Work out the finished part from the listing and answer in its coordinate system (mm). A direction names the side the tool comes from. Give positions to 0.01 mm unless a question says otherwise; leave off trailing zeros. Order: outer loops, then holes, each group sorted by start corner. A loop starts at its lowest first (then second) coordinate and runs counter-clockwise, first axis right, second up.
```python
from build123d import *

# Parameters (mm, degrees)
SKETCH001_W     = 100
SKETCH001_H     = 132
PAD_DEPTH       = 2.5
SKETCH002_R     = 3.5
SKETCH002_R_2   = 1.75
PAD001_DEPTH    = 4
PAD002_DEPTH    = 2.5
SKETCH004_R     = 3
HOLE_DEPTH      = 25
CHAMFER_1_ANGLE = 49
CHAMFER_1_SIZE  = 1
CHAMFER_2_ANGLE = 49
CHAMFER_2_SIZE  = 1
CHAMFER_3_ANGLE = 49
CHAMFER_3_SIZE  = 1
CHAMFER_4_ANGLE = 49
CHAMFER_4_SIZE  = 1
SKETCH005_W     = 10
SKETCH005_H     = 5
PAD003_DEPTH    = 12.5
FILLET_R        = 3.5
FILLET001_R     = 0.75


with BuildPart() as part:
    # Sketch001 → Pad (new body)
    with BuildSketch(Plane.XY):
        with Locations((50, 66)):
            Rectangle(SKETCH001_W, SKETCH001_H)
    extrude(amount=PAD_DEPTH)

    # Sketch002 (on Face6 of Pad) → Pad001 (join)
    with BuildSketch(Plane.XY.offset(2.5)):
        with Locations((76.5, 10)):
            Circle(SKETCH002_R)
        with Locations((76.5, 10)):
            Circle(SKETCH002_R_2, mode=Mode.SUBTRACT)
        with Locations((18.5, 10)):
            Circle(SKETCH002_R)
        with Locations((18.5, 10)):
            Circle(SKETCH002_R_2, mode=Mode.SUBTRACT)
        with Locations((18.5, 59)):
            Circle(SKETCH002_R)
        with Locations((18.5, 59)):
            Circle(SKETCH002_R_2, mode=Mode.SUBTRACT)
        with Locations((76.5, 59)):
            Circle(SKETCH002_R)
        with Locations((76.5, 59)):
            Circle(SKETCH002_R_2, mode=Mode.SUBTRACT)
        with Locations((87.1, 77.3)):
            Circle(SKETCH002_R)
        with Locations((87.1, 77.3)):
            Circle(SKETCH002_R_2, mode=Mode.SUBTRACT)
        with Locations((17.5, 77.3)):
            Circle(SKETCH002_R)
        with Locations((17.5, 77.3)):
            Circle(SKETCH002_R_2, mode=Mode.SUBTRACT)
        with Locations((17.5, 121.3)):
            Circle(SKETCH002_R)
        with Locations((17.5, 121.3)):
            Circle(SKETCH002_R_2, mode=Mode.SUBTRACT)
        with Locations((87.1, 121.3)):
            Circle(SKETCH002_R)
        with Locations((87.1, 121.3)):
            Circle(SKETCH002_R_2, mode=Mode.SUBTRACT)
    extrude(amount=PAD001_DEPTH)

    # Sketch003 → Pad002 (join)
    with BuildSketch(Plane.XY):
        with BuildLine():
            Line((-7.5, 102), (0, 102))
            Line((0, 102), (0, 87))
            Line((0, 87), (-7.5, 87))
            ThreePointArc((-7.5, 102), (-15.00002, 94.5), (-7.5, 87))
        make_face()
        with BuildLine():
            Line((-7.5, 45), (0, 45))
            Line((0, 45), (0, 30))
            Line((0, 30), (-7.5, 30))
            ThreePointArc((-7.5, 45), (-15.00002, 37.5), (-7.5, 30))
        make_face()
        with BuildLine():
            Line((100, 102), (107.5, 102))
            ThreePointArc((107.5, 87), (114.99998, 94.5), (107.5, 102))
            Line((107.5, 87), (100, 87))
            Line((100, 87), (100, 102))
        make_face()
        with BuildLine():
            Line((100, 45), (107.5, 45))
            ThreePointArc((107.5, 30), (114.99998, 37.5), (107.5, 45))
            Line((107.5, 30), (100, 30))
            Line((100, 30), (100, 45))
        make_face()
    extrude(amount=PAD002_DEPTH)

    # Sketch004 (on Face18 of Pad002) → Hole (cut)
    with BuildSketch(Plane.XY.offset(2.5)):
        with Locations((-7.5, 94.5)):
            Circle(SKETCH004_R)
        with Locations((107.5, 94.5)):
            Circle(SKETCH004_R)
        with Locations((107.5, 37.5)):
            Circle(SKETCH004_R)
        with Locations((-7.5, 37.5)):
            Circle(SKETCH004_R)
    extrude(amount=-HOLE_DEPTH, mode=Mode.SUBTRACT)

    # Chamfer 1
    chamfer_1_edges = [part.edges().sort_by_distance(p)[0] for p in [
        (104.5, 94.5, 2.5),
    ]]
    chamfer_1_side = part.faces().sort_by_distance((103.75, 87.212132, 2.5))[0]
    chamfer(chamfer_1_edges, length=CHAMFER_1_SIZE, angle=CHAMFER_1_ANGLE, reference=chamfer_1_side)

    # Chamfer 2
    chamfer_2_edges = [part.edges().sort_by_distance(p)[0] for p in [
        (104.5, 37.5, 2.5),
    ]]
    chamfer_2_side = part.faces().sort_by_distance((103.75, 30.212132, 2.5))[0]
    chamfer(chamfer_2_edges, length=CHAMFER_2_SIZE, angle=CHAMFER_2_ANGLE, reference=chamfer_2_side)

    # Chamfer 3
    chamfer_3_edges = [part.edges().sort_by_distance(p)[0] for p in [
        (-10.5, 37.5, 2.5),
    ]]
    chamfer_3_side = part.faces().sort_by_distance((-3.75, 44.787868, 2.5))[0]
    chamfer(chamfer_3_edges, length=CHAMFER_3_SIZE, angle=CHAMFER_3_ANGLE, reference=chamfer_3_side)

    # Chamfer 4
    chamfer_4_edges = [part.edges().sort_by_distance(p)[0] for p in [
        (-10.5, 94.5, 2.5),
    ]]
    chamfer_4_side = part.faces().sort_by_distance((-3.75, 101.787868, 2.5))[0]
    chamfer(chamfer_4_edges, length=CHAMFER_4_SIZE, angle=CHAMFER_4_ANGLE, reference=chamfer_4_side)

    # Sketch005 → Pad003 (join)
    with BuildSketch(Plane.XY):
        with Locations((-5, 66)):
            Rectangle(SKETCH005_W, SKETCH005_H)
        with Locations((-5, 76)):
            Rectangle(SKETCH005_W, SKETCH005_H)
        with Locations((-5, 56)):
            Rectangle(SKETCH005_W, SKETCH005_H)
    extrude(amount=PAD003_DEPTH)

    # Fillet
    fillet_edges = [part.edges().sort_by_distance(p)[0] for p in [
        (0, 56, 12.5),
        (-10, 56, 12.5),
        (-10, 66, 12.5),
        (0, 66, 12.5),
        (-10, 76, 12.5),
        (0, 76, 12.5),
    ]]
    fillet(fillet_edges, radius=FILLET_R)

    # Fillet001
    fillet001_edges = [part.edges().sort_by_distance(p)[0] for p in [
        (-5, 53.5, 12.5),
        (-5, 58.5, 12.5),
        (-5, 63.5, 12.5),
        (-5, 68.5, 12.5),
        (-5, 73.5, 12.5),
        (-5, 78.5, 12.5),
    ]]
    fillet(fillet001_edges, radius=FILLET001_R)


solid = part.part
```
1. The part is cut by section C-C (y = 10). Write down the section's boundary in (x, z).
Findings below:
outline: (0, 0) - (100, 0) - (100, 2.5) - (80, 2.5) - (80, 6.5) - (78.25, 6.5) - (78.25, 2.5) - (74.75, 2.5) - (74.75, 6.5) - (73, 6.5) - (73, 2.5) - (22, 2.5) - (22, 6.5) - (20.25, 6.5) - (20.25, 2.5) - (16.75, 2.5) - (16.75, 6.5) - (15, 6.5) - (15, 2.5) - (0, 2.5) - close
2. The mould has two halves that part along X. Classify faces 4 (the face through (-9, 56.02, 11.45)), 5 (the face through (-5, 53.5, 6)), 6 (the face through (-1, 56.02, 11.45)), 7 (the face through (0, 56, 6)): pulls with the +X half, pulls with the -X half, needs draft (parallel to the pull), parting line crosses it, or undercut.
Findings below:
face 4: pulls with the -X half
face 5: needs draft
face 6: pulls with the +X half
face 7: undercut
3. Straight lines are drawn through the part: probe 1 along Z at (x, y) = (8, 106); probe 2 along X at (y, z) = (75.5, 9.25); probe 3 along X at (y, z) = (13, 3). For each, find the intervals that lie inside material, in ascending order.
Findings below:
probe 1: z = 0 to 2.5
probe 2: x = -9.99 to -0.01
probe 3: x = 16.7 to 20.3, 74.7 to 78.3
4. The part is cut by section B-B (x = 76.5). Write down the section's boundary in (y, z), then the cut area to 3 significant figures.
Findings below:
outline: (0, 0) - (132, 0) - (132, 2.5) - (62.5, 2.5) - (62.5, 6.5) - (60.75, 6.5) - (60.75, 2.5) - (57.25, 2.5) - (57.25, 6.5) - (55.5, 6.5) - (55.5, 2.5) - (13.5, 2.5) - (13.5, 6.5) - (11.75, 6.5) - (11.75, 2.5) - (8.25, 2.5) - (8.25, 6.5) - (6.5, 6.5) - (6.5, 2.5) - (0, 2.5) - close
area: 358 mm2
5. Which of the six approach directions +Z, -Z, +X, -X, +Y, -Y give full straight-line access (tool end or side, diameter ignored) to faces 1 (the face through (-5, 73.5, 6)), 2 (the face through (17.272, 79.035, 4.472)), 3 (the face through (77, 61, 6.5))?
Findings below:
face 1: +Z, -Z, -X
face 2: +Z
face 3: +Z, +X, +Y, -Y
6. The part is cut by section A-A (y = 94.5). Write down the section's boundary in (x, z).
Findings below:
outline: (-15, 0) - (-10.5, 0) - (-10.5, 1.35) - (-11.5, 2.5) - (-15, 2.5) - close; (-4.5, 0) - (104.5, 0) - (104.5, 1.35) - (103.5, 2.5) - (-3.5, 2.5) - (-4.5, 1.35) - close; (110.5, 0) - (115, 0) - (115, 2.5) - (111.5, 2.5) - (110.5, 1.35) - close
7. Given P1, Ø1.8, axis at x = 76.5, y = 9.5, coming from the +Z side; P2, Ø4.5, axis at x = -4.5, z = 6.5, coming from the -Y side; P3, Ø3, axis at x = -2.5, z = 2, coming from the -Y side; P4, Ø2, axis at x = 76, y = 84.5, coming from the -Z side, each flat-ended and moving along its own axis, determine where each tip first touches the part or whether it passes through.
Findings below:
P1: stops at z = 2.5
P2: stops at y = 53.5
P3: stops at y = 30
P4: stops at z = 0
